from build123d import *

# Parameters (mm, degrees)
F0_W     = 117.930185
F0_H     = 107.323121
F1_DEPTH = 76.2
F2_R     = 39.627537
F3_DEPTH = 76.2
F4_R     = 6.35
F5_R     = 6.35
F6_R     = 4.388135
F7_DEPTH = 12.7
F8_R     = 1.851713
F9_DEPTH = 152.4


with BuildPart() as f1:
    # F0 (on Front) → F1 (new body)
    with BuildSketch(Plane.XZ):
        with Locations((1.745266, -15.826897)):
            Rectangle(F0_W, F0_H)
    extrude(amount=F1_DEPTH)

    # F2 (on face) → F3 (cut)
    with BuildSketch(Plane.XZ.offset(76.2)):
        with Locations((0, -16.006619)):
            Circle(F2_R)
    extrude(amount=-F3_DEPTH, mode=Mode.SUBTRACT)

    # F4
    f4_edges = [f1.edges().sort_by_distance(p)[0] for p in [
        (1.745267, 0, 37.834663),
        (-39.627537, 0, -16.006619),
    ]]
    fillet(f4_edges, radius=F4_R)

    # F5
    f5_edges = [f1.edges().sort_by_distance(p)[0] for p in [
        (60.710359, 0, -19.001898),
        (-57.219826, -41.275, 37.834663),
        (-57.219826, -1.859872, 35.974791),
        (-57.219826, -76.2, -15.826898),
        (-57.219826, 0, -19.001898),
        (-57.219826, -38.1, -69.488458),
    ]]
    fillet(f5_edges, radius=F5_R)

    # F6 (on face) → F7 (join)
    with BuildSketch(Plane(origin=(-57.219826, 0, 0), x_dir=(0, -1, 0), z_dir=(-1, 0, 0))):
        with Locations((11.499761, 21.451753)):
            Circle(F6_R)
    extrude(amount=F7_DEPTH)

    # F8 (on face) → F9 (cut)
    with BuildSketch(Plane(origin=(-69.919826, 0, 0), x_dir=(0, -1, 0), z_dir=(-1, 0, 0))):
        with Locations((11.499761, 21.451753)):
            Circle(F8_R)
    extrude(amount=-F9_DEPTH, mode=Mode.SUBTRACT)


solid = f1.part
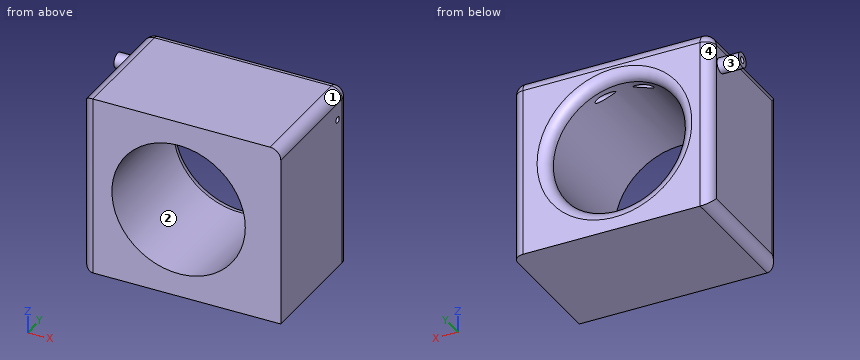
The model under review builds one solid part; all positions refer to its coordinate system, in mm. Face numbers are marked on the shaded views. Give positions to 0.01 mm unless a question says otherwise; leave off trailing zeros. Loops run counter-clockwise (first coordinate to the right, second up) from the corner with the lowest first, then second, coordinate; pieces in that order, holes last. Notation, with made-up numbers: (-7.5, 20.25) -> (19.5, 20.25) arc R12 cw to (19.5, 37.25) -> close; hole circle Ø8 at (-20.5, -12.5). An arc over 180 degrees is marked (long way). Write each question's results on one line, items separated by ' | '.
1) Insertion check: pin 1 Ø5 at (y, z) = (-18.5, -1.5) entering from -X; pin 2 Ø3 at (y, z) = (-11.5, 21.45) entering from -X. Each pin has a flat end and moves straight along its axis. Give the tip position at first contact, or say it passes through.
Conclusion:
pin 1: stops at x = -57.22 | pin 2: passes through
2) Take a section at C-C, the plane x = -24. Count the separate pieces of the cut face and the enclosed holes in it, plus the area to 3 significant figures.
Conclusion:
separate pieces: 2 | enclosed holes: 1 | area: 3,330 mm^2
3) Take a section at D-D, the plane x = -62. Give the boundary of the cut face in (y, z), plus the area to 3 significant figures.
Conclusion:
outline: circle Ø8.78 at (-11.5, 21.45); hole circle Ø3.7 at (-11.5, 21.45) | area: 49.7 mm^2
4) Take a section at B-B, the plane y = -47.5. Give the boundary of the cut face in (x, z).
Conclusion:
outline: (-57.22, -63.14) arc R6.35 ccw to (-50.87, -69.49) -> (60.71, -69.49) -> (60.71, 31.48) arc R6.35 ccw to (54.36, 37.83) -> (-50.87, 37.83) arc R6.35 ccw to (-57.22, 31.48) -> close; hole circle Ø79.26 at (0, -16.01)
5) Take a section at A-A, the plane x = 0. Give the boundary of the cut face in (y, z).
Conclusion:
outline: (-76.2, -69.49) -> (0, -69.49) -> (0, -61.98) arc R6.35 ccw to (-6.35, -55.63) -> (-76.2, -55.63) -> close; (-76.2, 23.62) -> (-6.35, 23.62) arc R6.35 ccw to (0, 29.97) -> (0, 31.48) arc R6.35 ccw to (-6.35, 37.83) -> (-76.2, 37.83) -> close
6) For line 1 along Z through (x, y) = (0, -22); line 2 along X through (y, z) = (-61.5, -15.5); line 3 along Z through (x, y) = (-29.5, -24.5), list the stretches that pass through material, from the lowest coordinate up. Write a range as from..to.
Conclusion:
line 1: z = -69.49..-55.63, 23.62..37.83 | line 2: x = -57.22..-39.62, 39.62..60.71 | line 3: z = -69.49..-42.47, 10.45..37.83
7) Draft analysis for pull direction X (two halves, no side actions). For the marked faces 1, 2, 3 and 4, state which applies: pulls with the +X half, pulls with the -X half, needs draft (parallel to the pull), parting line crosses it, or undercut.
Conclusion:
face 1: pulls with the +X half | face 2: undercut | face 3: needs draft | face 4: pulls with the -X half
